```python
from build123d import *

# Parameters (mm, degrees)
F1_DEPTH = 63.5
F2_DEPTH = 25.4
F3_DEPTH = 7.9375
F4_R     = 6.35


with BuildPart() as f1:
    # F0 (on Front) → F1 (new body, symmetric)
    with BuildSketch(Plane.XZ):
        Polygon((-41.275, 9.525), (-41.275, -9.525), (41.275, -9.525), (41.275, 9.525), (22.225, 9.525), align=None)
    extrude(amount=F1_DEPTH, both=True)

    # F0 (on Front) → F2 (join, symmetric)
    with BuildSketch(Plane.XZ):
        with BuildLine():
            Line((22.225, 9.525), (41.275, 9.525))
            Line((41.275, 9.525), (41.275, 27.0002))
            ThreePointArc((41.275, 27.0002), (44.060295, 35.982141), (51.438812, 41.812288))
            Line((51.438812, 41.812288), (51.438812, 61.455068))
            ThreePointArc((51.438812, 61.455068), (30.511505, 49.586616), (22.225, 27.0002))
            Line((22.225, 27.0002), (22.225, 9.525))
        make_face()
        with BuildLine():
            ThreePointArc((54.452364, 61.82086), (52.941612, 61.670722), (51.438812, 61.455068))
            Line((51.438812, 61.455068), (51.438812, 41.812288))
            ThreePointArc((51.438812, 41.812288), (54.245372, 42.60721), (57.15, 42.8752))
            Line((57.15, 42.8752), (85.725, 42.8752))
            Line((85.725, 42.8752), (85.725, 61.9252))
            Line((85.725, 61.9252), (57.15, 61.9252))
            add(Edge.make_bspline(
                [(54.452364, 61.82086), (55.352208, 61.866143), (56.251535, 61.90101), (57.15, 61.9252)],
                knots=[109.319651, 109.319651, 109.319651, 109.319651, 111.504536, 111.504536, 111.504536, 111.504536], degree=3))
        make_face()
    extrude(amount=F2_DEPTH, both=True)

    # F0 (on Front) → F3 (join, symmetric)
    with BuildSketch(Plane.XZ):
        with BuildLine():
            add(Edge.make_bspline(
                [(-41.275, 9.525), (-36.986678, 30.729489), (7.384144, 58.294379), (51.438812, 61.630741)],
                knots=[0, 0, 0, 0, 106.881788, 106.881788, 106.881788, 106.881788], degree=3))
            Line((-41.275, 9.525), (22.225, 9.525))
            Line((22.225, 9.525), (22.225, 27.0002))
            ThreePointArc((22.225, 27.0002), (30.511505, 49.586616), (51.438812, 61.455068))
            Line((51.438812, 61.455068), (51.438812, 61.630741))
        make_face()
    extrude(amount=F3_DEPTH, both=True)

    # F4
    f4_edges = [f1.edges().sort_by_distance(p)[0] for p in [
        (-41.275, -63.5, 0),
        (41.275, -63.5, 0),
        (41.275, 63.5, 0),
        (-41.275, 63.5, 0),
    ]]
    fillet(f4_edges, radius=F4_R)


solid = f1.part
```
Here's how the part is built. I have some questions about the finished solid (model axes, mm). A direction names the side the tool comes from. Coordinates: 2 decimals unless noted, no trailing zeros. Loops run counter-clockwise (first coordinate to the right, second up) from the corner with the lowest first, then second, coordinate; pieces in that order, holes last. Notation, with made-up numbers: M -25.5,23.25 L 22.5,23.25 A25 ccw 22.5,57.25 Z; hole C 75,-34 d11. An arc over 180 degrees is marked long. One line per item, written item: value.
1. Imagine slicing it at B-B (x = 74.5). List the corners of the cut face in (y, z) for me, and give its area (3 significant figures).
Geometry says:
outline: M -25.4,42.88 L 25.4,42.88 L 25.4,61.93 L -25.4,61.93 Z
area: 968 mm2
2. Please list where these lines run through material, in increasing order: probe 1 along Y at (x, z) = (25.5, 38); probe 2 along X at (y, z) = (11.5, 6) (3 decimals); probe 3 along Y at (x, z) = (-4, 39).
Geometry says:
probe 1: y = -25.4 to 25.4
probe 2: x = -41.275 to 41.275
probe 3: y = -7.94 to 7.94
3. Imagine slicing it at A-A (y = -54). List the corners of the cut face in (x, z) for me (3 decimals).
Geometry says:
outline: M -41.275,-9.525 L 41.275,-9.525 L 41.275,9.525 L -41.275,9.525 Z
4. On a 3-axis mill with a long thin cutter (end or side, diameter ignored), from which of +Z, -Z, +X, -X, +Y, -Y can I reach the whole of each face in a straight line? I mean faces 1 (the flat face through (22.225, 17, 18)), 2 (the flat face through (46, 25.4, 42)), 3 (the flat face through (1, -36, 9.525)), 4 (the flat face through (46, -25.4, 42)). Say none if no direction works.
Geometry says:
face 1: +Z, -X, +Y
face 2: +Z, +X, -X, +Y
face 3: +Z, -X, -Y
face 4: +Z, +X, -X, -Y
5. Will these pins go through, and if not, where does the flat tip stop? pin 1 Ø8 at (x, z) = (37, 6.5) entering from -Y; pin 2 Ø1.5 at (x, z) = (-4.5, 25) entering from -Y; pin 3 Ø1 at (x, y) = (57.5, -19.5) entering from -Z; pin 4 Ø10 at (x, y) = (26.5, -37.5) entering from +Z (3 decimals).
Geometry says:
pin 1: stops at y = -63.5
pin 2: stops at y = -7.94
pin 3: stops at z = 42.87
pin 4: stops at z = 9.525
